from build123d import *

# Parameters (mm, degrees)
BOSS_EXTRUDE1_DEPTH = 25.4
FILLET1_R           = 2.0955
FILLET2_R           = 1.397
FILLET3_R           = 0.6985
CUT_EXTRUDE1_REACH  = 4.794
SKETCH4_R           = 2.0828
CUT_EXTRUDE2_REACH  = 4.794
SKETCH5_R           = 2.0828


with BuildPart() as part:
    # Sketch3 → Boss-Extrude1 (new body, symmetric)
    with BuildSketch(Plane(origin=(0, 0, 0), x_dir=(1, 0, 0), z_dir=(0, 1, 0))):
        Polygon((1.397, -1.397), (65.278, -1.397), (65.278, 1.397), (-1.397, 1.397), (-1.397, -65.278), (1.397, -65.278), align=None)
    extrude(amount=BOSS_EXTRUDE1_DEPTH, both=True)

    # Fillet1
    fillet1_edges = [part.edges().sort_by_distance(p)[0] for p in [
        (-1.397, 0, -1.397),
    ]]
    fillet(fillet1_edges, radius=FILLET1_R)

    # Fillet2
    fillet2_edges = [part.edges().sort_by_distance(p)[0] for p in [
        (1.397, 0, 1.397),
    ]]
    fillet(fillet2_edges, radius=FILLET2_R)

    # Fillet3
    fillet3_edges = [part.edges().sort_by_distance(p)[0] for p in [
        (65.278, 25.4, 0),
        (0, 25.4, 65.278),
        (0, -25.4, 65.278),
        (65.278, -25.4, 0),
    ]]
    fillet(fillet3_edges, radius=FILLET3_R)

    # Sketch4 → Cut-Extrude1 (cut, up to next)
    with BuildSketch(Plane(origin=(1.397, 0, 0), x_dir=(0, 0, -1), z_dir=(1, 0, 0)), mode=Mode.PRIVATE) as cut_extrude1_sk1:
        with Locations((-52.578, -6.35)):
            Circle(SKETCH4_R)
    cut_extrude1_tool1 = extrude(cut_extrude1_sk1.sketch, amount=-CUT_EXTRUDE1_REACH, mode=Mode.PRIVATE) & part.part
    add(cut_extrude1_tool1.solids().sort_by_distance((1.397, -6.35, 52.578))[0], mode=Mode.SUBTRACT)
    # Sketch4 → Cut-Extrude1 (cut, up to next)
    with BuildSketch(Plane(origin=(1.397, 0, 0), x_dir=(0, 0, -1), z_dir=(1, 0, 0)), mode=Mode.PRIVATE) as cut_extrude1_sk2:
        with Locations((-27.178, 6.35)):
            Circle(SKETCH4_R)
    cut_extrude1_tool2 = extrude(cut_extrude1_sk2.sketch, amount=-CUT_EXTRUDE1_REACH, mode=Mode.PRIVATE) & part.part
    add(cut_extrude1_tool2.solids().sort_by_distance((1.397, 6.35, 27.178))[0], mode=Mode.SUBTRACT)
    # Sketch4 → Cut-Extrude1 (cut, up to next)
    with BuildSketch(Plane(origin=(1.397, 0, 0), x_dir=(0, 0, -1), z_dir=(1, 0, 0)), mode=Mode.PRIVATE) as cut_extrude1_sk3:
        with Locations((-27.178, -12.7)):
            Circle(SKETCH4_R)
    cut_extrude1_tool3 = extrude(cut_extrude1_sk3.sketch, amount=-CUT_EXTRUDE1_REACH, mode=Mode.PRIVATE) & part.part
    add(cut_extrude1_tool3.solids().sort_by_distance((1.397, -12.7, 27.178))[0], mode=Mode.SUBTRACT)
    # Sketch4 → Cut-Extrude1 (cut, up to next)
    with BuildSketch(Plane(origin=(1.397, 0, 0), x_dir=(0, 0, -1), z_dir=(1, 0, 0)), mode=Mode.PRIVATE) as cut_extrude1_sk4:
        with Locations((-52.578, 12.7)):
            Circle(SKETCH4_R)
    cut_extrude1_tool4 = extrude(cut_extrude1_sk4.sketch, amount=-CUT_EXTRUDE1_REACH, mode=Mode.PRIVATE) & part.part
    add(cut_extrude1_tool4.solids().sort_by_distance((1.397, 12.7, 52.578))[0], mode=Mode.SUBTRACT)

    # Sketch5 → Cut-Extrude2 (cut, up to next)
    with BuildSketch(Plane.XY.offset(1.397), mode=Mode.PRIVATE) as cut_extrude2_sk1:
        with Locations((27.178, 12.7)):
            Circle(SKETCH5_R)
    cut_extrude2_tool1 = extrude(cut_extrude2_sk1.sketch, amount=-CUT_EXTRUDE2_REACH, mode=Mode.PRIVATE) & part.part
    add(cut_extrude2_tool1.solids().sort_by_distance((27.178, 12.7, 1.397))[0], mode=Mode.SUBTRACT)
    # Sketch5 → Cut-Extrude2 (cut, up to next)
    with BuildSketch(Plane.XY.offset(1.397), mode=Mode.PRIVATE) as cut_extrude2_sk2:
        with Locations((27.178, -6.35)):
            Circle(SKETCH5_R)
    cut_extrude2_tool2 = extrude(cut_extrude2_sk2.sketch, amount=-CUT_EXTRUDE2_REACH, mode=Mode.PRIVATE) & part.part
    add(cut_extrude2_tool2.solids().sort_by_distance((27.178, -6.35, 1.397))[0], mode=Mode.SUBTRACT)
    # Sketch5 → Cut-Extrude2 (cut, up to next)
    with BuildSketch(Plane.XY.offset(1.397), mode=Mode.PRIVATE) as cut_extrude2_sk3:
        with Locations((52.578, -12.7)):
            Circle(SKETCH5_R)
    cut_extrude2_tool3 = extrude(cut_extrude2_sk3.sketch, amount=-CUT_EXTRUDE2_REACH, mode=Mode.PRIVATE) & part.part
    add(cut_extrude2_tool3.solids().sort_by_distance((52.578, -12.7, 1.397))[0], mode=Mode.SUBTRACT)
    # Sketch5 → Cut-Extrude2 (cut, up to next)
    with BuildSketch(Plane.XY.offset(1.397), mode=Mode.PRIVATE) as cut_extrude2_sk4:
        with Locations((52.578, 6.35)):
            Circle(SKETCH5_R)
    cut_extrude2_tool4 = extrude(cut_extrude2_sk4.sketch, amount=-CUT_EXTRUDE2_REACH, mode=Mode.PRIVATE) & part.part
    add(cut_extrude2_tool4.solids().sort_by_distance((52.578, 6.35, 1.397))[0], mode=Mode.SUBTRACT)


solid = part.part
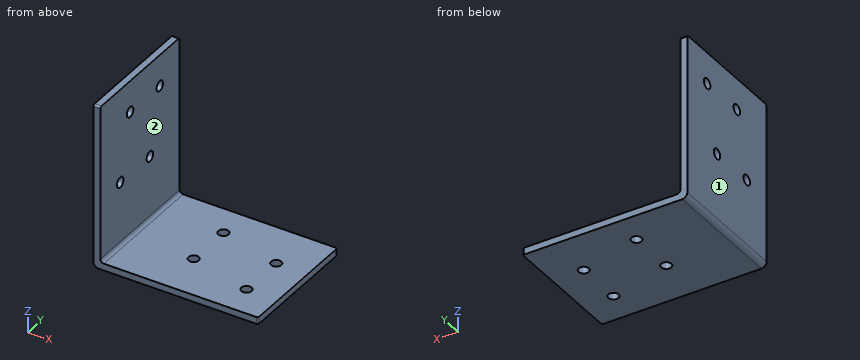
Geometry check sheet. Reference: the model listing, model coordinates, mm. Face numbers are marked on the shaded views. A direction names the side the tool comes from. Give positions to 0.01 mm unless a question says otherwise; leave off trailing zeros. Order: outer loops, then holes, each group sorted by start corner. A loop starts at its lowest first (then second) coordinate and runs counter-clockwise, first axis right, second up. Notation, with made-up numbers: (58.5, -35) - (89.5, -35) arc R27 ccw to (89.5, -9) - close; hole circle Ø3 at (38, 72). An arc over 180 degrees is marked (long way). Answer as a JSON object with one key per item and string values.
(1) Tool access check on the marked faces 1 and 2. Record the directions out of +Z, -Z, +X, -X, +Y, -Y that give a thin tool (end or side, any length) a straight path to the whole face; none if there is none.
Report:
{"face 1": "+Z, -Z, -X, +Y, -Y", "face 2": "+Z, +X, +Y, -Y"}
(2) Material ranges on line 1 (Z direction, x = 34.5, y = 8); line 2 (Z direction, x = 0, y = 12), recorded low to high.
Report:
{"line 1": "-1.4 to 1.4", "line 2": "-1.28 to 50.62, 54.54 to 65.28"}
(3) Cross-section at B-B (y = 21). Record the cut outline in (x, z), then the cut area to 3 significant figures.
Report:
{"outline": "(-1.4, 0.7) arc R2.1 ccw to (0.7, -1.4) - (65.28, -1.4) - (65.28, 1.4) - (2.79, 1.4) arc R1.4 cw to (1.4, 2.79) - (1.4, 65.28) - (-1.4, 65.28) - close", "area": "364 mm^2"}
(4) Depth check by flat-ended pin: pin 1 Ø5 at (y, z) = (-12.7, 27.178) entering from +X; pin 2 Ø3.5 at (x, y) = (52.578, 6.35) entering from -Z; pin 3 Ø1 at (x, y) = (14, 7) entering from +Z. Enter the tip coordinate at first touch or a pass-through.
Report:
{"pin 1": "x = 1.4", "pin 2": "through", "pin 3": "z = 1.4"}
(5) Cross-section at C-C (x = 57.5). Record the cut outline in (y, z).
Report:
{"outline": "(-25.4, -1.4) - (25.4, -1.4) - (25.4, 1.4) - (-25.4, 1.4) - close"}
(6) Cross-section at D-D (z = 40). Record the cut outline in (x, y), then the cut area to 3 significant figures.
Report:
{"outline": "(-1.4, -25.4) - (1.4, -25.4) - (1.4, 25.4) - (-1.4, 25.4) - close", "area": "142 mm^2"}
(7) Cross-section at A-A (y = 6.35). Record the cut outline in (x, z).
Report:
{"outline": "(-1.4, 0.7) arc R2.1 ccw to (0.7, -1.4) - (50.5, -1.4) - (50.5, 1.4) - (2.79, 1.4) arc R1.4 cw to (1.4, 2.79) - (1.4, 25.1) - (-1.4, 25.1) - close; (-1.4, 29.26) - (1.4, 29.26) - (1.4, 65.28) - (-1.4, 65.28) - close; (54.66, -1.4) - (65.28, -1.4) - (65.28, 1.4) - (54.66, 1.4) - close"}
